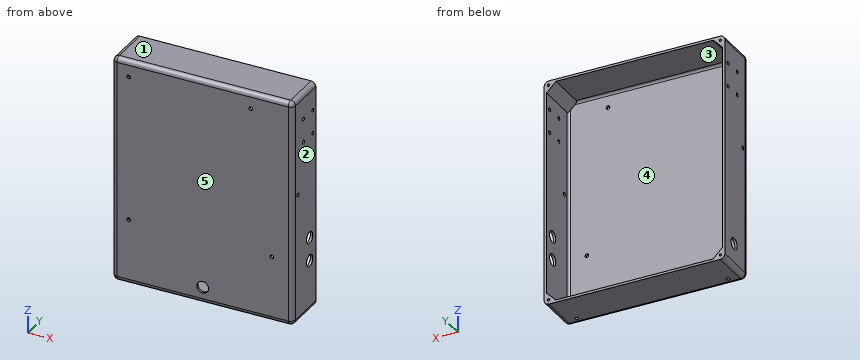
```python
from build123d import *

# Parameters (mm, degrees)
SKETCH1_W                           = 190.5
SKETCH1_H                           = 241.3
BOSS_EXTRUDE1_DEPTH                 = 44.45
FILLET1_R                           = 2.54
SHELL1_T                            = 2.54
HOLE_A_D                            = 4
BOSS_EXTRUDE3_REACH                 = 166.155
MIRROR3_COPY_1_REACH                = 166.155
COVER_HOLES_D                       = 2.64668
COVER_HOLES_DEPTH                   = 12.7
COVER_HOLES_TIP                     = 0.795142892
HOLE_FOR_WIRING_D                   = 12.7
HOLE_TO_OUTSIDE_WIRING_D            = 12.7
HOLE_TO_OUTSIDE_WIRING_DEPTH        = 2.54
HOLE_TO_OUTSIDE_WIRING_TIP          = 3.815464931
F_9_64_0_15_DIAMETER_HOLE1_D        = 3.81
F_9_64_0_14063_DIAMETER_HOLE2_D     = 3.572002
F_9_64_0_14063_DIAMETER_HOLE2_DEPTH = 2.54
F_9_64_0_14063_DIAMETER_HOLE2_TIP   = 1.073137666
ANTENNA_HOLES_D                     = 12.7
ANTENNA_HOLES_DEPTH                 = 2.54
ANTENNA_HOLES_TIP                   = 3.815464931
F_1_8_0_15_DIAMETER_HOLE1_D         = 3.81


with BuildPart() as part:
    # Sketch1 → Boss-Extrude1 (new body)
    with BuildSketch(Plane(origin=(0, 0, 0), x_dir=(1, 0, 0), z_dir=(0, 1, 0))):
        Rectangle(SKETCH1_W, SKETCH1_H)
    extrude(amount=BOSS_EXTRUDE1_DEPTH)

    # Fillet1
    fillet1_edges = [part.edges().sort_by_distance(p)[0] for p in [
        (0, 0, -120.65),
        (95.25, 0, 0),
        (0, 0, 120.65),
        (-95.25, 0, 0),
        (-95.25, 22.225, -120.65),
        (95.25, 22.225, -120.65),
        (95.25, 22.225, 120.65),
        (-95.25, 22.225, 120.65),
    ]]
    fillet(fillet1_edges, radius=FILLET1_R)

    # Shell1
    shell1_openings = [part.faces().sort_by_distance(p)[0] for p in [
        (0, 44.45, 0),
    ]]
    offset(amount=SHELL1_T, openings=shell1_openings, kind=Kind.INTERSECTION)

    # Hole A (through all)
    with Locations(Plane(origin=(0, 0, 0), x_dir=(1, 0, 0), z_dir=(0, 1, 0))):
        with Locations((-80.01, 52.07), (74.91000004, 52.07), (-80.01, -105.41), (52.07, -105.41)):
            Hole(HOLE_A_D / 2)

    # Boss-Extrude3: up to this face of the body (flat: up to its plane)
    boss_extrude3_end = Plane(part.part.faces().sort_by_distance((0.0094902, 0, -0.030642085))[0])
    # Sketch25 → Boss-Extrude3 (add, up to the picked face)
    with BuildSketch(Plane(origin=(0, 44.45, 0), x_dir=(1, 0, 0), z_dir=(0, 1, 0)), mode=Mode.PRIVATE) as boss_extrude3_sk1:
        Polygon((85.09, 120.65), (95.25, 110.49), (95.25, 120.65), align=None)
    boss_extrude3_tool1 = split(extrude(boss_extrude3_sk1.sketch, amount=-BOSS_EXTRUDE3_REACH, mode=Mode.PRIVATE), bisect_by=boss_extrude3_end, keep=Keep.BOTH, mode=Mode.PRIVATE)
    boss_extrude3 = boss_extrude3_tool1.solids().sort_by(Axis((91.863333, 44.45, -117.263333), (0, -1, 0)))[0]
    add(boss_extrude3)

    # Mirror2: Boss-Extrude3 across plane
    add(boss_extrude3.mirror(Plane.XY))

    # Mirror3: Boss-Extrude3 across plane
    add(boss_extrude3.mirror(Plane(origin=(0, 0, 0), x_dir=(0, 0, 1), z_dir=(1, 0, 0))))

    # Mirror3 copy 1: up to this face of the body (flat: up to its plane)
    mirror3_copy_1_end = Plane(part.part.faces().sort_by_distance((-0.0094902, 0, 0.030642085))[0])
    # Mirror3 copy 1 sketch → Mirror3 copy 1 (add, up to the picked face)
    with BuildSketch(Plane(origin=(0, 44.45, 0), x_dir=(-1, 0, 0), z_dir=(0, 1, 0)), mode=Mode.PRIVATE) as mirror3_copy_1_sk1:
        Polygon((85.09, 120.65), (95.25, 110.49), (95.25, 120.65), align=None)
    mirror3_copy_1_tool1 = split(extrude(mirror3_copy_1_sk1.sketch, amount=-MIRROR3_COPY_1_REACH, mode=Mode.PRIVATE), bisect_by=mirror3_copy_1_end, keep=Keep.BOTH, mode=Mode.PRIVATE)
    add(mirror3_copy_1_tool1.solids().sort_by(Axis((-91.863333, 44.45, 117.263333), (0, -1, 0)))[0])

    # Cover Holes
    with Locations(Plane(origin=(0, 44.45, 0), x_dir=(1, 0, 0), z_dir=(0, 1, 0))):
        with Locations((-93.0275, 118.4275), (-93.0275, -118.4275), (93.0275, -118.4275), (93.0275, 118.4275)):
            Hole(COVER_HOLES_D / 2, depth=COVER_HOLES_DEPTH)
            with Locations((0, 0, -(COVER_HOLES_DEPTH + COVER_HOLES_TIP / 2))):  # 118° drill point
                Cone(0, COVER_HOLES_D / 2, COVER_HOLES_TIP, mode=Mode.SUBTRACT)

    # Hole for wiring (through all)
    with Locations(Plane(origin=(0, 0, 0), x_dir=(1, 0, 0), z_dir=(0, 1, 0))):
        with Locations((0, 105.41)):
            Hole(HOLE_FOR_WIRING_D / 2)

    # Hole to outside wiring
    with Locations(Plane.ZY.offset(97.79)):
        with Locations((-97.79, 25.4)):
            Hole(HOLE_TO_OUTSIDE_WIRING_D / 2, depth=HOLE_TO_OUTSIDE_WIRING_DEPTH)
            with Locations((0, 0, -(HOLE_TO_OUTSIDE_WIRING_DEPTH + HOLE_TO_OUTSIDE_WIRING_TIP / 2))):  # 118° drill point
                Cone(0, HOLE_TO_OUTSIDE_WIRING_D / 2, HOLE_TO_OUTSIDE_WIRING_TIP, mode=Mode.SUBTRACT)

    # 9/64 (0.15) Diameter Hole1 (through all)
    with Locations(Plane(origin=(97.79, 0, 0), x_dir=(0, 0, -1), z_dir=(1, 0, 0))):
        with Locations((-17.145, 7.62)):
            Hole(F_9_64_0_15_DIAMETER_HOLE1_D / 2)

    # 9/64 (0.14063) Diameter Hole2
    with Locations(Plane(origin=(0, 0, -123.19), x_dir=(-1, 0, 0), z_dir=(0, 0, -1))):
        with Locations((-81.915, 7.62), (81.915, 7.62)):
            Hole(F_9_64_0_14063_DIAMETER_HOLE2_D / 2, depth=F_9_64_0_14063_DIAMETER_HOLE2_DEPTH)
            with Locations((0, 0, -(F_9_64_0_14063_DIAMETER_HOLE2_DEPTH + F_9_64_0_14063_DIAMETER_HOLE2_TIP / 2))):  # 118° drill point
                Cone(0, F_9_64_0_14063_DIAMETER_HOLE2_D / 2, F_9_64_0_14063_DIAMETER_HOLE2_TIP, mode=Mode.SUBTRACT)

    # Antenna Holes
    with Locations(Plane(origin=(97.79, 0, 0), x_dir=(0, 0, -1), z_dir=(1, 0, 0))):
        with Locations((67.31, 31.75), (41.91, 31.75)):
            Hole(ANTENNA_HOLES_D / 2, depth=ANTENNA_HOLES_DEPTH)
            with Locations((0, 0, -(ANTENNA_HOLES_DEPTH + ANTENNA_HOLES_TIP / 2))):  # 118° drill point
                Cone(0, ANTENNA_HOLES_D / 2, ANTENNA_HOLES_TIP, mode=Mode.SUBTRACT)

    # 1/8 (0.15) Diameter Hole1 (through all)
    with Locations(Plane(origin=(97.79, 0, 0), x_dir=(0, 0, -1), z_dir=(1, 0, 0))):
        with Locations((-95.25, 38.1), (-69.85, 38.1), (-95.25, 19.05), (-69.85, 19.05)):
            Hole(F_1_8_0_15_DIAMETER_HOLE1_D / 2)


solid = part.part
```
Could you check a few things on this model? Use its own coordinates, in mm. Face numbers are marked on the shaded views. A direction names the side the tool comes from. Give positions to 0.01 mm unless a question says otherwise; leave off trailing zeros. Loops run counter-clockwise (first coordinate to the right, second up) from the corner with the lowest first, then second, coordinate; pieces in that order, holes last. Notation, with made-up numbers: (17.5, -31) - (60.5, -31) arc R13 cw to (60.5, -24) - close; hole circle Ø6 at (52.5, 32.5). An arc over 180 degrees is marked (long way). Use one line per item in the form item = value.
1. I want a section at B-B (z = -41.91). Please give me the cut outline in (x, y).
Response values:
outline = (-97.79, 2.54) arc R5.08 ccw to (-92.71, -2.54) - (92.71, -2.54) arc R5.08 ccw to (97.79, 2.54) - (97.79, 25.4) - (95.25, 25.4) - (95.25, 2.54) arc R2.54 cw to (92.71, 0) - (-92.71, 0) arc R2.54 cw to (-95.25, 2.54) - (-95.25, 44.45) - (-97.79, 44.45) - close; (95.25, 38.1) - (97.79, 38.1) - (97.79, 44.45) - (95.25, 44.45) - close
2. I need wall thicknesses on probe 1 along Z at (x, y) = (-74, 42.5); probe 2 along X at (y, z) = (42, 45.5); probe 3 along Y at (x, z) = (-96, 69). Which ranges of each line are inside material? Lowest first, please.
Response values:
probe_1 = -123.19 to -120.65, 120.65 to 123.19
probe_2 = -97.79 to -95.25, 95.25 to 97.79
probe_3 = -1.33 to 17.35, 20.75 to 36.4, 39.8 to 44.45
3. I want a section at A-A (x = 0). Please give me the cut outline in (y, z), and give its area (3 significant figures).
Response values:
outline = (-2.54, -118.11) arc R5.08 ccw to (2.54, -123.19) - (44.45, -123.19) - (44.45, -120.65) - (2.54, -120.65) arc R2.54 cw to (0, -118.11) - (0, -111.76) - (-2.54, -111.76) - close; (-2.54, -99.06) - (0, -99.06) - (0, 118.11) arc R2.54 cw to (2.54, 120.65) - (44.45, 120.65) - (44.45, 123.19) - (2.54, 123.19) arc R5.08 ccw to (-2.54, 118.11) - close
area = 811 mm²
4. I'm going to push flat-ended pins straight in: pin 1 Ø2.5 at (x, z) = (93.03, -118.43) entering from +Y; pin 2 Ø8 at (x, z) = (77.5, -61.5) entering from +Y. Where does each tip first touch, or does it pass through?
Response values:
pin_1 = 31.71
pin_2 = 0
5. Thinking about a two-plate mould opening in Z: for the marked faces 1, 2 and 3, which applies, released by +Z, released by -Z, zero draft, split by the parting line, or undercut?
Response values:
face_1 = released by +Z
face_2 = zero draft
face_3 = undercut
6. I want a section at C-C (x = 69.5). Please give me the cut outline in (y, z).
Response values:
outline = (-2.54, -118.11) arc R5.08 ccw to (2.54, -123.19) - (44.45, -123.19) - (44.45, -120.65) - (2.54, -120.65) arc R2.54 cw to (0, -118.11) - (0, 118.11) arc R2.54 cw to (2.54, 120.65) - (44.45, 120.65) - (44.45, 123.19) - (2.54, 123.19) arc R5.08 ccw to (-2.54, 118.11) - close
7. I want a section at D-D (z = -15.5). Please give me the cut outline in (x, y), and give its area (3 significant figures).
Response values:
outline = (-97.79, 2.54) arc R5.08 ccw to (-92.71, -2.54) - (92.71, -2.54) arc R5.08 ccw to (97.79, 2.54) - (97.79, 44.45) - (95.25, 44.45) - (95.25, 2.54) arc R2.54 cw to (92.71, 0) - (-92.71, 0) arc R2.54 cw to (-95.25, 2.54) - (-95.25, 44.45) - (-97.79, 44.45) - close
area = 714 mm²
8. On a 3-axis mill with a long thin cutter (end or side, diameter ignored), from which of +Z, -Z, +X, -X, +Y, -Y can I reach the whole of each face in a straight line? I mean the marked faces 4 and 5. Say none if no direction works.
Response values:
face_4 = +Y
face_5 = +Z, -Z, +X, -X, -Y
